from build123d import *

# Parameters (mm, degrees)
F0_W      = 50.8
F0_H      = 13.97
F1_DEPTH  = 19.05
F3_DEPTH  = 19.05
F5_DEPTH  = 25.4
F6_R      = 3.2385
F7_DEPTH  = 25.4
F8_R      = 4.8475114841
F9_DEPTH  = 12.7
F10_W     = 20.32
F10_H     = 19.05
F11_DEPTH = 10.16
F12_W     = 14.8905639175
F12_H     = 6.35
F13_DEPTH = 25.4


with BuildPart() as f1:
    # F0 (on Front) → F1 (new body)
    with BuildSketch(Plane.XZ):
        with Locations((0, -6.985)):
            Rectangle(F0_W, F0_H)
    extrude(amount=-F1_DEPTH)

    # F2 (on face) → F3 (cut)
    with BuildSketch(Plane.XZ):
        with BuildLine():
            ThreePointArc((-10.668, 0), (0, -10.668), (10.668, 0))
            Line((10.668, 0), (-10.668, 0))
        make_face()
    extrude(amount=-F3_DEPTH, mode=Mode.SUBTRACT)

    # F4 (on face) → F5 (cut)
    with BuildSketch(Plane.XZ):
        Polygon((-25.4, -3.81), (-25.4, -13.97), (-10.16, -13.97), align=None)
        Polygon((25.4, -13.97), (25.4, -3.81), (10.16, -13.97), align=None)
    extrude(amount=-F5_DEPTH, mode=Mode.SUBTRACT)

    # F6 (on face) → F7 (cut)
    with BuildSketch(Plane.XY):
        with Locations((-17.4625, 9.525)):
            Circle(F6_R)
        with Locations((17.4625, 9.525)):
            Circle(F6_R)
    extrude(amount=-F7_DEPTH, mode=Mode.SUBTRACT)

    # F8 (on face) → F9 (cut)
    with BuildSketch(Plane(origin=(0, 0, -13.97), x_dir=(1, 0, 0), z_dir=(0, 0, -1))):
        with Locations((-17.4625, -9.525)):
            Circle(F8_R)
        with Locations((17.4625, -9.525)):
            Circle(F8_R)
    extrude(amount=-F9_DEPTH, mode=Mode.SUBTRACT)

    # F10 (on face) → F11 (join)
    with BuildSketch(Plane(origin=(0, 0, -13.97), x_dir=(1, 0, 0), z_dir=(0, 0, -1))):
        with Locations((0, -9.525)):
            Rectangle(F10_W, F10_H)
    extrude(amount=F11_DEPTH)

    # F12 (on face) → F13 (cut)
    with BuildSketch(Plane(origin=(-10.16, 0, 0), x_dir=(0, -1, 0), z_dir=(-1, 0, 0))):
        with Locations((-11.6047180412, -17.2086453915)):
            Rectangle(F12_W, F12_H)
    extrude(amount=-F13_DEPTH, mode=Mode.SUBTRACT)


solid = f1.part
Could you check a few things on this model? Use its own coordinates, in mm. A direction names the side the tool comes from. Round coordinates to 2 decimals unless told otherwise and drop trailing zeros. Order: outer loops, then holes, each group sorted by start corner. A loop starts at its lowest first (then second) coordinate and runs counter-clockwise, first axis right, second up. Notation, with made-up numbers: M -33.5,-36 L -11.5,-36 A17 ccw -11.5,-19 Z; hole C 46,16.5 d5. An arc over 180 degrees is marked long. One line per item, written item: value.
(1) If we mould it in two halves opening along Z, with no side actions, what happens to faces 1 (the flat face through (0, 12, -14.034)), 2 (the flat face through (10.16, 8, -21)), 3 (the flat face through (21, 11, -1.27))? For each: released by +Z, released by -Z, zero draft, split by the parting line, or undercut.
Ans:
face 1: undercut
face 2: zero draft
face 3: released by -Z
(2) Imagine slicing it at D-D (x = -17). Write out the boundary of the cut face in (y, z).
Ans:
outline: M 0,-9.41 L 4.7,-9.41 L 4.7,-1.27 L 6.32,-1.27 L 6.32,0 L 0,0 Z; M 12.73,-1.27 L 14.35,-1.27 L 14.35,-9.41 L 19.05,-9.41 L 19.05,0 L 12.73,0 Z
(3) Imagine slicing it at A-A (y = 16.25). Write out the boundary of the cut face in (x, z).
Ans:
outline: M -25.4,-3.81 L -10.16,-13.97 L -10.16,-14.03 L 10.16,-14.03 L 10.16,-13.97 L 25.4,-3.81 L 25.4,0 L 10.67,0 A10.67 cw -10.67,0 L -25.4,0 Z; M -10.16,-24.13 L 10.16,-24.13 L 10.16,-20.38 L -10.16,-20.38 Z
(4) Imagine slicing it at C-C (x = 0). Write out the boundary of the cut face in (y, z), and give its area (3 significant figures).
Ans:
outline: M 0,-24.13 L 19.05,-24.13 L 19.05,-20.38 L 4.16,-20.38 L 4.16,-14.03 L 19.05,-14.03 L 19.05,-10.67 L 0,-10.67 Z
area: 162 mm^2
(5) Which directions (+Z, -Z, +X, -X, +Y, -Y) give clear straight access to the entire face, cutting with the end or side of a thin tool? Please do faces 4 (the flat face through (-25.4, 9, -2)), 5 (the cylindrical face through (12.62, 9.31, -5.7)), 6 (the flat face through (0, 19.05, -22)), 7 (the flat face through (-10.16, 8, -21)), 8 (the flat face through (0, 4.159, -17)).
Ans:
face 4: +Z, -Z, -X, +Y, -Y
face 5: -Z
face 6: +Z, -Z, +X, -X, +Y
face 7: -Z, -X, +Y, -Y
face 8: +X, -X, +Y
(6) I need wall thicknesses on line 1 along Z through (x, y) = (-20.5, 13); line 2 along Y through (x, z) = (0, -14.75); line 3 along X through (y, z) = (14.5, -3.75). Which ranges of each line are inside material? Lowest first, please. Write a range as from..to.
Ans:
line 1: z = -1.27..0
line 2: y = 0..4.16
line 3: x = -25.4..-9.99, 9.99..25.4
(7) I'm going to push flat-ended pins straight in: P1, Ø5, axis at y = 7, z = -21, coming from the -X side; P2, Ø3, axis at y = 13, z = -21, coming from the +X side; P3, Ø10.5, axis at x = -17.46, y = 9.52, coming from the -Z side. Where does each tip first touch, or does it pass through?
Ans:
P1: stops at x = -10.16
P2: stops at x = 10.16
P3: stops at z = -12.6
